from build123d import *

# Parameters (mm, degrees)
BOSS_EXTRUDE1_OUTLINE_W  = 4.7752
BOSS_EXTRUDE1_OUTLINE_H  = 50.8
BOSS_EXTRUDE1_DEPTH      = 50.8
F_0_257_DIAMETER_HOLE1_D = 6.5278
FILLET1_R                = 0.381
LPATTERN1_COUNT          = 2
LPATTERN1_PITCH          = 25.4
LPATTERN1_COUNT_DIR2     = 2
LPATTERN1_PITCH_DIR2     = 25.4


# Read off the part's stored shape, not the designer's step: Boss-Extrude1
with BuildPart() as part:
    # Boss-Extrude1 outline → Boss-Extrude1 (new body)
    with BuildSketch(Plane.YZ):
        with Locations((2.3876, 25.4)):
            Rectangle(BOSS_EXTRUDE1_OUTLINE_W, BOSS_EXTRUDE1_OUTLINE_H)
    extrude(amount=BOSS_EXTRUDE1_DEPTH)

    # F (0.257) Diameter Hole1 (through all)
    with Locations(Plane(origin=(0, 4.7752, 0), x_dir=(1, 0, 0), z_dir=(0, 1, 0))):
        with Locations((38.1, -38.1)):
            f_0_257_diameter_hole1 = Hole(F_0_257_DIAMETER_HOLE1_D / 2)

    # Fillet1
    fillet1_edges = [part.edges().sort_by_distance(p)[0] for p in [
        (50.8, 4.7752, 25.4),
        (0, 4.7752, 25.4),
        (50.8, 0, 25.4),
        (0, 0, 25.4),
    ]]
    fillet(fillet1_edges, radius=FILLET1_R)

    # LPattern1: F _0.257_ Diameter Hole1 2 × 2
    with Locations(*[(-i * LPATTERN1_PITCH, 0, -j * LPATTERN1_PITCH_DIR2) for i in range(LPATTERN1_COUNT) for j in range(LPATTERN1_COUNT_DIR2) if (i, j) != (0, 0)]):
        add(f_0_257_diameter_hole1, mode=Mode.SUBTRACT)


solid = part.part
The listing builds one solid part. Answer for the finished solid, in the listing's coordinates (mm). Coordinates: 2 decimals unless noted, no trailing zeros. Loops run counter-clockwise (first coordinate to the right, second up) from the corner with the lowest first, then second, coordinate; pieces in that order, holes last. Notation, with made-up numbers: (-15.5, -29) -> (-4.5, -29) arc R36 ccw to (-4.5, 6) -> close; hole circle Ø5 at (37.5, 68.5). An arc over 180 degrees is marked (long way). Answer in a Markdown table with one row per item. Add a question column.
1. The part is cut by section A-A, the plane z = 38.1. Write down the section's boundary in (x, y), then the cut area to 3 significant figures.
2. The part is cut by section C-C, the plane y = 1.2. Write down the section's boundary in (x, z), then the cut area to 3 significant figures.
3. Consider line 1 (Z direction, x = 12.7, y = 2.8); line 2 (X direction, y = 1.7, z = 36). Determine where each line is inside the solid, lowest interval first. Write a range as [from, to].
4. The part is cut by section D-D, the plane z = 14. Write down the section's boundary in (x, y), then the cut area to 3 significant figures.
5. Determine the mould class of faces 1 (the flat face through (25, 2, 50.8)), 2 (the flat face through (50.8, 2, 26)), 3 (the flat face through (25, 2, 0)), 4 (the cylindrical face through (13.408, 2.354, 41.286)) for opening direction Z: +Z half, -Z half, draft (parallel to the pull), parting line (faces both ways), or undercut.
6. The part is cut by section B-B, the plane x = 12.7. Write down the section's boundary in (y, z), then the cut area to 3 significant figures.
Answer below:
| question | item | result |
|---|---|---|
| 1 | outline | (0, 0.38) arc R0.38 ccw to (0.38, 0) -> (9.44, 0) -> (9.44, 4.78) -> (0.38, 4.78) arc R0.38 ccw to (0, 4.39) -> close; (15.96, 0) -> (34.84, 0) -> (34.84, 4.78) -> (15.96, 4.78) -> close; (41.36, 0) -> (50.42, 0) arc R0.38 ccw to (50.8, 0.38) -> (50.8, 4.39) arc R0.38 ccw to (50.42, 4.78) -> (41.36, 4.78) -> close |
| 1 | area | 180 mm2 |
| 2 | outline | (0, 0) -> (50.8, 0) -> (50.8, 50.8) -> (0, 50.8) -> close; hole circle Ø6.53 at (12.7, 12.7); hole circle Ø6.53 at (12.7, 38.1); hole circle Ø6.53 at (38.1, 12.7); hole circle Ø6.53 at (38.1, 38.1) |
| 2 | area | 2,450 mm2 |
| 3 | line 1 | [0, 9.44], [15.96, 34.84], [41.36, 50.8] |
| 3 | line 2 | [0, 10.2], [15.2, 35.6], [40.6, 50.8] |
| 4 | outline | (0, 0.38) arc R0.38 ccw to (0.38, 0) -> (9.71, 0) -> (9.71, 4.78) -> (0.38, 4.78) arc R0.38 ccw to (0, 4.39) -> close; (15.69, 0) -> (35.11, 0) -> (35.11, 4.78) -> (15.69, 4.78) -> close; (41.09, 0) -> (50.42, 0) arc R0.38 ccw to (50.8, 0.38) -> (50.8, 4.39) arc R0.38 ccw to (50.42, 4.78) -> (41.09, 4.78) -> close |
| 4 | area | 185 mm2 |
| 5 | face 1 | +Z half |
| 5 | face 2 | draft |
| 5 | face 3 | -Z half |
| 5 | face 4 | undercut |
| 6 | outline | (0, 0) -> (4.78, 0) -> (4.78, 9.44) -> (0, 9.44) -> close; (0, 15.96) -> (4.78, 15.96) -> (4.78, 34.84) -> (0, 34.84) -> close; (0, 41.36) -> (4.78, 41.36) -> (4.78, 50.8) -> (0, 50.8) -> close |
| 6 | area | 180 mm2 |
